from build123d import *

# Parameters (mm, degrees)
SKETCH_W  = 50
SKETCH_H  = 10
SKETCH_R  = 3
PAD_DEPTH = 10


with BuildPart() as part:
    # Sketch → Pad (new body)
    with BuildSketch(Plane.YZ):
        with Locations((20, 0)):
            Rectangle(SKETCH_W, SKETCH_H)
        Circle(SKETCH_R, mode=Mode.SUBTRACT)
    extrude(amount=PAD_DEPTH)


solid = part.part
Geometry check sheet. Reference: the model listing, model coordinates, mm. Coordinates: 2 decimals unless noted, no trailing zeros. Order: outer loops, then holes, each group sorted by start corner. A loop starts at its lowest first (then second) coordinate and runs counter-clockwise, first axis right, second up. Notation, with made-up numbers: (-5, 41) - (-1, 41) arc R24 ccw to (-1, 73) - close; hole circle Ø6 at (-25, 35.25). An arc over 180 degrees is marked (long way). Answer in a Markdown table with one row per item. Add a question column.
1) Cross-section at B-B, the plane y = 0. Record the cut outline in (x, z).
2) Cross-section at A-A, the plane z = 0. Record the cut outline in (x, y).
3) Cross-section at C-C, the plane x = 1. Record the cut outline in (y, z), then the cut area to 3 significant figures.
4) Material ranges on line 1 along Z through (x, y) = (7.5, 0); line 2 along Y through (x, z) = (5.75, 2); line 3 along Y through (x, z) = (1.75, 0.5), recorded low to high. Write a range as [from, to].
5) Release check for a two-part mould opening along Z. For faces 1 (the flat face through (5, 20, 5)), 2 (the cylindrical face through (5, -3, 0)), 3 (the flat face through (5, -5, 0)) record: +Z half, -Z half, draft (parallel to the pull), parting line (faces both ways), or undercut.
Check result:
| question | item | result |
|---|---|---|
| 1 | outline | (0, -5) - (10, -5) - (10, -3) - (0, -3) - close; (0, 3) - (10, 3) - (10, 5) - (0, 5) - close |
| 2 | outline | (0, -5) - (10, -5) - (10, -3) - (0, -3) - close; (0, 3) - (10, 3) - (10, 45) - (0, 45) - close |
| 3 | outline | (-5, -5) - (45, -5) - (45, 5) - (-5, 5) - close; hole circle Ø6 at (0, 0) |
| 3 | area | 472 mm² |
| 4 | line 1 | z = [-5, -3], [3, 5] |
| 4 | line 2 | y = [-5, -2.24], [2.24, 45] |
| 4 | line 3 | y = [-5, -2.96], [2.96, 45] |
| 5 | face 1 | +Z half |
| 5 | face 2 | undercut |
| 5 | face 3 | draft |
